from build123d import *

# Parameters (mm, degrees)
SKETCH_1_W          = 40
SKETCH_1_H          = 30
EXTRUDE_1_DEPTH     = 5
SKETCH_2_R          = 2
CUT_EXTRUDE_1_DEPTH = 5
SKETCH_3_R          = 3
CUT_EXTRUDE_2_DEPTH = 2.5
SKETCH_5_W          = 40
SKETCH_5_H          = 30
SKETCH_5_R          = 2
EXTRUDE_2_DEPTH     = 3
SKETCH_3_2_R        = 3
CUT_EXTRUDE_3_DEPTH = 3
SKETCH_9_W          = 40
SKETCH_9_H          = 30
SKETCH_9_R          = 2
EXTRUDE_4_DEPTH     = 2
SKETCH_8_R          = 2
CUT_EXTRUDE_5_DEPTH = 10
CUT_EXTRUDE_START   = 10
SKETCH_8_4_R        = 2
CUT_EXTRUDE_6_DEPTH = 10
CUT_EXTRUDE_7_DEPTH = 3
CUT_EXTRUDE_8_DEPTH = 3


with BuildPart() as part:
    # Sketch 1 → Extrude 1 (new body)
    with BuildSketch(Plane.XY):
        with Locations((20, 15)):
            Rectangle(SKETCH_1_W, SKETCH_1_H)
    extrude(amount=EXTRUDE_1_DEPTH)

    # Sketch 2 → Cut-Extrude 1 (cut)
    with BuildSketch(Plane.XY.offset(5)):
        with Locations((3, 25)):
            Circle(SKETCH_2_R)
        with Locations((3, 5)):
            Circle(SKETCH_2_R)
        with Locations((26.7, 15)):
            Circle(SKETCH_2_R)
    extrude(amount=-CUT_EXTRUDE_1_DEPTH, mode=Mode.SUBTRACT)

    # Sketch 3 → Cut-Extrude 2 (cut)
    with BuildSketch(Plane.XY.offset(5)):
        with Locations((26.7, 15)):
            Circle(SKETCH_3_R)
        Polygon((3, 22), (6, 22), (6, 30), (0, 30), (0, 22), align=None)
        Polygon((3, 8), (0, 8), (0, 0), (6, 0), (6, 8), align=None)
    extrude(amount=-CUT_EXTRUDE_2_DEPTH, mode=Mode.SUBTRACT)

    # Sketch 5 → Extrude 2 (add)
    with BuildSketch(Plane(origin=(0, 0, 0), x_dir=(-1, 0, 0), z_dir=(0, 0, -1))):
        with Locations((-20, 15)):
            Rectangle(SKETCH_5_W, SKETCH_5_H)
        with Locations(Location((-26.7, 15, 0), (0, 0, 180))):
            Circle(SKETCH_5_R, mode=Mode.SUBTRACT)
        with Locations(Location((-3, 25, 0), (0, 0, 180))):
            Circle(SKETCH_5_R, mode=Mode.SUBTRACT)
        with Locations(Location((-3, 5, 0), (0, 0, 180))):
            Circle(SKETCH_5_R, mode=Mode.SUBTRACT)
    extrude(amount=EXTRUDE_2_DEPTH)

    # Sketch 3_2 → Cut-Extrude 3 (cut)
    with BuildSketch(Plane.XY.offset(5)):
        with Locations((26.7, 15)):
            Circle(SKETCH_3_2_R)
        Polygon((3, 22), (6, 22), (6, 30), (0, 30), (0, 22), align=None)
        Polygon((3, 8), (0, 8), (0, 0), (6, 0), (6, 8), align=None)
    extrude(amount=-CUT_EXTRUDE_3_DEPTH, mode=Mode.SUBTRACT)

    # Sketch 9 → Extrude 4 (add)
    with BuildSketch(Plane(origin=(0, 0, -3), x_dir=(-1, 0, 0), z_dir=(0, 0, -1))):
        with Locations((-20, 15)):
            Rectangle(SKETCH_9_W, SKETCH_9_H)
        with Locations(Location((-26.7, 15, 0), (0, 0, 180))):
            Circle(SKETCH_9_R, mode=Mode.SUBTRACT)
        with Locations(Location((-3, 25, 0), (0, 0, 180))):
            Circle(SKETCH_9_R, mode=Mode.SUBTRACT)
        with Locations(Location((-3, 5, 0), (0, 0, 180))):
            Circle(SKETCH_9_R, mode=Mode.SUBTRACT)
    extrude(amount=EXTRUDE_4_DEPTH)

    # Sketch 8 → Cut-Extrude 5 (cut)
    with BuildSketch(Plane(origin=(0, 0, -3), x_dir=(-1, 0, 0), z_dir=(0, 0, -1))):
        with Locations((-37, 25)):
            Circle(SKETCH_8_R)
        with Locations((-37, 5)):
            Circle(SKETCH_8_R)
        with Locations((-10, 15)):
            Circle(SKETCH_8_R)
    extrude(amount=-CUT_EXTRUDE_5_DEPTH, mode=Mode.SUBTRACT)

    # Sketch 8_4 → Cut-Extrude 6 (cut)
    with BuildSketch(Plane(origin=(0, 0, -3), x_dir=(-1, 0, 0), z_dir=(0, 0, -1)).offset(CUT_EXTRUDE_START)):
        with Locations((-37, 25)):
            Circle(SKETCH_8_4_R)
        with Locations((-37, 5)):
            Circle(SKETCH_8_4_R)
        with Locations((-10, 15)):
            Circle(SKETCH_8_4_R)
    extrude(amount=-CUT_EXTRUDE_6_DEPTH, mode=Mode.SUBTRACT)

    # Sketch 11 → Cut-Extrude 7 (cut)
    with BuildSketch(Plane(origin=(0, 0, -5), x_dir=(-1, 0, 0), z_dir=(0, 0, -1))):
        Polygon((-37, 22), (-40, 22), (-40, 30), (-34, 30), (-34, 22), align=None)
        Polygon((-37, 8), (-40, 8), (-40, 0), (-34, 0), (-34, 8), align=None)
        Polygon((-10, 18), (-7, 18), (-7, 12), (-13, 12), (-13, 18), align=None)
    extrude(amount=-CUT_EXTRUDE_7_DEPTH, mode=Mode.SUBTRACT)

    # Sketch 12 → Cut-Extrude 8 (cut)
    with BuildSketch(Plane.XY.offset(5)):
        Polygon((26.7, 18), (29.7, 18), (29.7, 12), (23.7, 12), (23.7, 18), align=None)
    extrude(amount=-CUT_EXTRUDE_8_DEPTH, mode=Mode.SUBTRACT)


solid = part.part
For this review, take the finished solid that the model builds, in its own axes (mm). A direction names the side the tool comes from. Round coordinates to 2 decimals unless told otherwise and drop trailing zeros. Order: outer loops, then holes, each group sorted by start corner. A loop starts at its lowest first (then second) coordinate and runs counter-clockwise, first axis right, second up. Notation, with made-up numbers: (-16.75, 7.5) -> (-6.75, 7.5) arc R29 ccw to (-6.75, 40.5) -> close; hole circle Ø8 at (0.5, 34). An arc over 180 degrees is marked (long way). Put each result on its own line as item: value.
Q1. For probe 1 along Y at (x, z) = (37, 1.75); probe 2 along Y at (x, z) = (10, 1.5); probe 3 along Y at (x, z) = (28, 2.75), list the stretches that pass through material, from the lowest coordinate up. Write a range as [from, to].
Check result:
probe 1: [0, 3], [7, 23], [27, 30]
probe 2: [0, 13], [17, 30]
probe 3: [0, 12], [18, 30]
Q2. Add section B-B on z = -1.25. Write out the cut boundary in (x, y), plus the area to 3 significant figures.
Check result:
outline: (0, 0) -> (40, 0) -> (40, 30) -> (0, 30) -> close; hole circle Ø4 at (3, 5); hole circle Ø4 at (3, 25); hole circle Ø4 at (10, 15); hole circle Ø4 at (26.7, 15); hole circle Ø4 at (37, 5); hole circle Ø4 at (37, 25)
area: 1,120 mm2
Q3. Add section C-C on x = 26.7. Write out the cut boundary in (y, z).
Check result:
outline: (0, -5) -> (13, -5) -> (13, 2) -> (12, 2) -> (12, 5) -> (0, 5) -> close; (17, -5) -> (30, -5) -> (30, 5) -> (18, 5) -> (18, 2) -> (17, 2) -> close
Q4. Add section D-D on y = 5. Write out the cut boundary in (x, z).
Check result:
outline: (0, -5) -> (1, -5) -> (1, 2) -> (0, 2) -> close; (5, -5) -> (34, -5) -> (34, -2) -> (35, -2) -> (35, 5) -> (6, 5) -> (6, 2) -> (5, 2) -> close; (39, -2) -> (40, -2) -> (40, 5) -> (39, 5) -> close
Q5. Mouldability with a two-part tool opening along X and no side actions: class faces 1 (the flat face through (6, 26, 4)), 2 (the flat face through (29, 15, 2)), 3 (the flat face through (36, 27, -2)), 4 (the cylindrical face through (39, 5, 1)) as pulls with the +X half, pulls with the -X half, needs draft (parallel to the pull), parting line crosses it, or undercut.
Check result:
face 1: pulls with the -X half
face 2: undercut
face 3: needs draft
face 4: undercut
Q6. Machinability: for faces 5 (the flat face through (2, 27, 2)), 6 (the flat face through (10, 12, -4)), 7 (the flat face through (34, 26, -4)), 8 (the flat face through (27, 18, 4)), 9 (the flat face through (34, 4, -4)), which of the approach directions +Z, -Z, +X, -X, +Y, -Y give a long, thin tool a straight path to every point of the face, cutting with its end or side? Answer none if there is none.
Check result:
face 5: +Z, -X, +Y
face 6: -Z
face 7: -Z, +X, +Y
face 8: +Z
face 9: -Z, +X, -Y
Q7. Insertion check: pin 1 Ø3 at (x, y) = (2, 26.5) entering from +Z; pin 2 Ø0.9 at (x, z) = (38.5, -3) entering from +Y; pin 3 Ø2.5 at (y, z) = (26.5, 4) entering from -X; pin 4 Ø2.5 at (x, y) = (10, 15) entering from -Z. Each pin has a flat end and moves straight along its axis. Give the tip position at first contact, or say it passes through.
Check result:
pin 1: z = 2
pin 2: y = 22
pin 3: x = 6
pin 4: through
Q8. Add section A-A on x = 3. Write out the cut boundary in (y, z).
Check result:
outline: (0, -5) -> (3, -5) -> (3, 2) -> (0, 2) -> close; (7, -5) -> (23, -5) -> (23, 2) -> (22, 2) -> (22, 5) -> (8, 5) -> (8, 2) -> (7, 2) -> close; (27, -5) -> (30, -5) -> (30, 2) -> (27, 2) -> close
